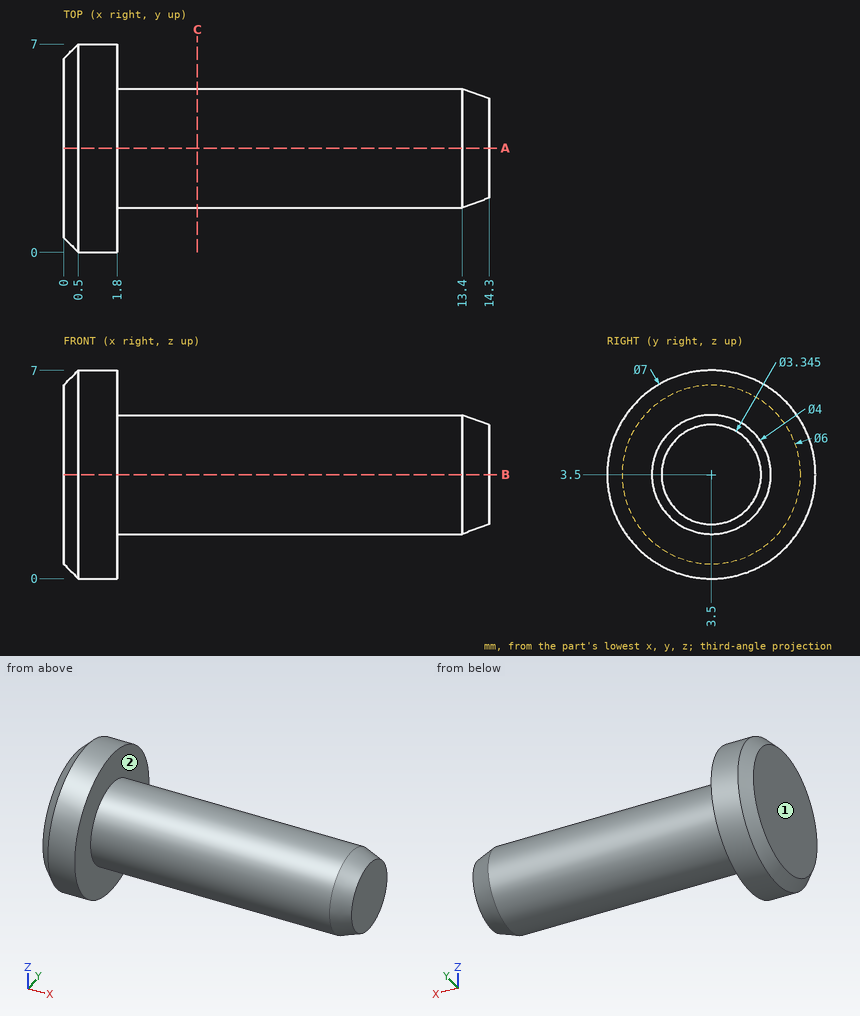
Input: dimensioned drawing with shaded views. Units: mm. Origin: part minimum x, y, z. A direction names the side the tool comes from. Give positions to 0.01 mm unless a question says otherwise; leave off trailing zeros. Write each loop counter-clockwise with the first axis right and the second up, starting at its lowest first coordinate (ties: lowest second). Pieces come first, ordered by that corner, then holes. Notation, with made-up numbers: M 37.5,21.5 L 58.5,21.5 A7 cw 58.5,32.5 Z; hole C 1,-4.75 d4. An arc over 180 degrees is marked long. Return JSON: item names as keys, results as strings. Group by question number.
1) Material intervals for line 1 along X through (y, z) = (1.5, 4.75); line 2 along Z through (x, y) = (4.5, 3.5); line 3 along Z through (x, y) = (9.75, 2), sorted ascending. Write a range as [from, to].
2) Cut plane C-C, the plane x = 4.5. Output: boundary loops of the cut face in (y, z).
3) Cut plane A-A, the plane y = 3.5. Output: boundary loops of the cut face in (x, z).
4) Pin query (flat end, axial travel): P1, Ø1.5, axis at x = 3.5, z = 5.5, coming from the +Y side; P2, Ø3, axis at x = 10.5, y = 1, coming from the +Z side; P3, Ø3, axis at x = 9, y = 1.5, coming from the +Z side. Return the tip coordinate at first contact, or that it passes through.
5) Set-up query: the marked faces 1 and 2. Return all of +Z, -Z, +X, -X, +Y, -Y with unobstructed straight access to the full face (end or side cutting, diameter ignored); none if empty.
Recorded:
{
 "1": {"line 1": "x = [0, 1.8]", "line 2": "z = [1.5, 5.5]", "line 3": "z = [2.18, 4.82]"},
 "2": {"outline": "C 3.5,3.5 d4"},
 "3": {"outline": "M 0,0.5 L 0.5,0 L 1.8,0 L 1.8,1.5 L 13.4,1.5 L 14.3,1.83 L 14.3,5.17 L 13.4,5.5 L 1.8,5.5 L 1.8,7 L 0.5,7 L 0,6.5 Z"},
 "4": {"P1": "stops at y = 5.06", "P2": "stops at z = 5.23", "P3": "stops at z = 5.44"},
 "5": {"face 1": "+Z, -Z, -X, +Y, -Y", "face 2": "+X"}
}
